Input: part model. Units: mm. Frame: model coordinates. A direction names the side the tool comes from. Give positions to 0.01 mm unless a question says otherwise; leave off trailing zeros. Write each loop counter-clockwise with the first axis right and the second up, starting at its lowest first coordinate (ties: lowest second). Pieces come first, ordered by that corner, then holes. Notation, with made-up numbers: (-23, 21) - (-12, 21) arc R17 cw to (-12, 41) - close; hole circle Ø6 at (27.25, -37). An arc over 180 degrees is marked (long way). Answer as CSV lines item,"result".
```python
from build123d import *

# Parameters (mm, degrees)
SKETCH1_W                 = 90
SKETCH1_H                 = 72
BOSS_EXTRUDE1_DEPTH       = 40
SHELL1_T                  = -2
SHELL1_THICKNESS_2_FACE_W = 86
SHELL1_THICKNESS_2_FACE_H = 38
SHELL1_THICKNESS_2_DEPTH  = 1
SHELL1_THICKNESS_3_FACE_W = 86
SHELL1_THICKNESS_3_FACE_H = 38
SHELL1_THICKNESS_3_DEPTH  = 1
SHELL1_THICKNESS_4_FACE_W = 66
SHELL1_THICKNESS_4_FACE_H = 38
SHELL1_THICKNESS_4_DEPTH  = 1.5
SKETCH2_R                 = 1.5
CUT_EXTRUDE1_DEPTH        = 2
CUT_EXTRUDE2_DEPTH        = 88
BOSS_EXTRUDE2_REACH       = 103.874
SKETCH4_W                 = 2
SKETCH4_H                 = 5
SKETCH5_R                 = 1.65
SKETCH5_W                 = 45
SKETCH5_H                 = 15
CUT_EXTRUDE3_DEPTH        = 3.5
CUT_EXTRUDE4_DEPTH        = 2.1
CUT_EXTRUDE5_REACH        = 106.862
SKETCH7_R                 = 2.55
SKETCH7_W                 = 10
SKETCH7_H                 = 10
SKETCH8_W                 = 16
SKETCH8_H                 = 9
SKETCH8_W_2               = 11
SKETCH8_H_2               = 7
CUT_EXTRUDE6_DEPTH        = 3
BOSS_EXTRUDE3_DEPTH       = 70
SKETCH10_R                = 1.65
SKETCH10_W                = 15.5
SKETCH10_H                = 9.5
CUT_EXTRUDE7_DEPTH        = 3
CUT_EXTRUDE8_DEPTH        = 2.1
FILLET3_R                 = 1
FILLET4_R                 = 0.5
FILLET5_R                 = 0.5
FILLET6_R                 = 0.5
FILLET7_R                 = 6
FILLET8_R                 = 4
FILLET9_R                 = 2
FILLET10_R                = 2


with BuildPart() as part:
    # Sketch1 → Boss-Extrude1 (new body)
    with BuildSketch(Plane(origin=(0, 0, 0), x_dir=(1, 0, 0), z_dir=(0, 1, 0))):
        Rectangle(SKETCH1_W, SKETCH1_H)
    extrude(amount=BOSS_EXTRUDE1_DEPTH)

    # Shell1
    shell1_openings = [part.faces().sort_by_distance(p)[0] for p in [
        (0, 40, 0),
    ]]
    offset(amount=SHELL1_T, openings=shell1_openings, kind=Kind.INTERSECTION)

    # Shell1 thickness 2 face (on inner face of the shell) → Shell1 thickness 2 (add)
    with BuildSketch(Plane(origin=(0, 21, 34), x_dir=(1, 0, 0), z_dir=(0, 0, 1))):
        Rectangle(SHELL1_THICKNESS_2_FACE_W, SHELL1_THICKNESS_2_FACE_H)
    extrude(amount=-SHELL1_THICKNESS_2_DEPTH)

    # Shell1 thickness 3 face (on inner face of the shell) → Shell1 thickness 3 (add)
    with BuildSketch(Plane(origin=(0, 21, -34), x_dir=(-1, 0, 0), z_dir=(0, 0, -1))):
        Rectangle(SHELL1_THICKNESS_3_FACE_W, SHELL1_THICKNESS_3_FACE_H)
    extrude(amount=-SHELL1_THICKNESS_3_DEPTH)

    # Shell1 thickness 4 face (on inner face of the shell) → Shell1 thickness 4 (add)
    with BuildSketch(Plane(origin=(43, 21, 0), x_dir=(0, 0, 1), z_dir=(1, 0, 0))):
        Rectangle(SHELL1_THICKNESS_4_FACE_W, SHELL1_THICKNESS_4_FACE_H)
    extrude(amount=-SHELL1_THICKNESS_4_DEPTH)

    # Sketch2 → Cut-Extrude1 (cut)
    with BuildSketch(Plane(origin=(0, 2, 0), x_dir=(1, 0, 0), z_dir=(0, 1, 0))):
        with Locations(Location((37.5, 27.5, 0), (0, 0, 270))):
            Circle(SKETCH2_R)
        with Locations(Location((-37.5, 27.5, 0), (0, 0, 270))):
            Circle(SKETCH2_R)
        with Locations(Location((-37.5, -27.5, 0), (0, 0, 270))):
            Circle(SKETCH2_R)
        with Locations(Location((37.5, -27.5, 0), (0, 0, 270))):
            Circle(SKETCH2_R)
    extrude(amount=-CUT_EXTRUDE1_DEPTH, mode=Mode.SUBTRACT)

    # Sketch3 → Cut-Extrude2 (cut)
    with BuildSketch(Plane(origin=(45, 0, 0), x_dir=(0, 0, -1), z_dir=(1, 0, 0))):
        Polygon((-30.5, 40), (-33.5, 37), (33.5, 37), (30.5, 40), align=None)
    extrude(amount=-CUT_EXTRUDE2_DEPTH, mode=Mode.SUBTRACT)

    # Sketch4 → Boss-Extrude2 (add, up to next)
    with BuildSketch(Plane.ZY.offset(-41.5), mode=Mode.PRIVATE) as boss_extrude2_sk1:
        Polygon((30.5, 40), (33, 37.5), (33, 40), align=None)
    boss_extrude2_tool1 = extrude(boss_extrude2_sk1.sketch, amount=BOSS_EXTRUDE2_REACH, mode=Mode.PRIVATE) - part.part
    # Sketch4 → Boss-Extrude2 (add, up to next)
    with BuildSketch(Plane.ZY.offset(-41.5), mode=Mode.PRIVATE) as boss_extrude2_sk2:
        Polygon((-33, 37.5), (-30.5, 40), (-33, 40), align=None)
    boss_extrude2_tool2 = extrude(boss_extrude2_sk2.sketch, amount=BOSS_EXTRUDE2_REACH, mode=Mode.PRIVATE) - part.part
    # Sketch4 → Boss-Extrude2 (add, up to next)
    with BuildSketch(Plane.ZY.offset(-41.5), mode=Mode.PRIVATE) as boss_extrude2_sk3:
        with Locations((-32, 34.5)):
            Rectangle(SKETCH4_W, SKETCH4_H)
    boss_extrude2_tool3 = extrude(boss_extrude2_sk3.sketch, amount=BOSS_EXTRUDE2_REACH, mode=Mode.PRIVATE) - part.part
    # Sketch4 → Boss-Extrude2 (add, up to next)
    with BuildSketch(Plane.ZY.offset(-41.5), mode=Mode.PRIVATE) as boss_extrude2_sk4:
        with Locations((32, 34.5)):
            Rectangle(SKETCH4_W, SKETCH4_H)
    boss_extrude2_tool4 = extrude(boss_extrude2_sk4.sketch, amount=BOSS_EXTRUDE2_REACH, mode=Mode.PRIVATE) - part.part
    add(boss_extrude2_tool1.solids().sort_by_distance((41.5, 39.166667, 32.166667))[0])
    add(boss_extrude2_tool2.solids().sort_by_distance((41.5, 39.166667, -32.166667))[0])
    add(boss_extrude2_tool3.solids().sort_by_distance((41.5, 34.5, -32))[0])
    add(boss_extrude2_tool4.solids().sort_by_distance((41.5, 34.5, 32))[0])

    # Sketch5 → Cut-Extrude3 (cut)
    with BuildSketch(Plane(origin=(45, 0, 0), x_dir=(0, 0, -1), z_dir=(1, 0, 0))):
        with Locations((0, 17)):
            Circle(SKETCH5_R)
        with Locations((0, 29.5)):
            Rectangle(SKETCH5_W, SKETCH5_H)
    extrude(amount=-CUT_EXTRUDE3_DEPTH, mode=Mode.SUBTRACT)

    # Sketch6 → Cut-Extrude4 (cut)
    with BuildSketch(Plane.ZY.offset(-41.5)):
        Polygon((3.117691454, 17), (1.558845727, 19.7), (-1.558845727, 19.7), (-3.117691454, 17), (-1.558845727, 14.3), (1.558845727, 14.3), align=None)
    extrude(amount=-CUT_EXTRUDE4_DEPTH, mode=Mode.SUBTRACT)

    # Sketch7 → Cut-Extrude5 (cut, up to next)
    with BuildSketch(Plane.ZY.offset(45), mode=Mode.PRIVATE) as cut_extrude5_sk1:
        with Locations((-22.5, 30)):
            Circle(SKETCH7_R)
    cut_extrude5_tool1 = extrude(cut_extrude5_sk1.sketch, amount=-CUT_EXTRUDE5_REACH, mode=Mode.PRIVATE) & part.part
    # Sketch7 → Cut-Extrude5 (cut, up to next)
    with BuildSketch(Plane.ZY.offset(45), mode=Mode.PRIVATE) as cut_extrude5_sk2:
        with Locations((-7.5, 30)):
            Circle(SKETCH7_R)
    cut_extrude5_tool2 = extrude(cut_extrude5_sk2.sketch, amount=-CUT_EXTRUDE5_REACH, mode=Mode.PRIVATE) & part.part
    # Sketch7 → Cut-Extrude5 (cut, up to next)
    with BuildSketch(Plane.ZY.offset(45), mode=Mode.PRIVATE) as cut_extrude5_sk3:
        with Locations((7.5, 30)):
            Circle(SKETCH7_R)
    cut_extrude5_tool3 = extrude(cut_extrude5_sk3.sketch, amount=-CUT_EXTRUDE5_REACH, mode=Mode.PRIVATE) & part.part
    # Sketch7 → Cut-Extrude5 (cut, up to next)
    with BuildSketch(Plane.ZY.offset(45), mode=Mode.PRIVATE) as cut_extrude5_sk4:
        with Locations((22.5, 30)):
            Circle(SKETCH7_R)
    cut_extrude5_tool4 = extrude(cut_extrude5_sk4.sketch, amount=-CUT_EXTRUDE5_REACH, mode=Mode.PRIVATE) & part.part
    # Sketch7 → Cut-Extrude5 (cut, up to next)
    with BuildSketch(Plane.ZY.offset(45), mode=Mode.PRIVATE) as cut_extrude5_sk5:
        with Locations((-4, 17)):
            Rectangle(SKETCH7_W, SKETCH7_H)
    cut_extrude5_tool5 = extrude(cut_extrude5_sk5.sketch, amount=-CUT_EXTRUDE5_REACH, mode=Mode.PRIVATE) & part.part
    add(cut_extrude5_tool1.solids().sort_by_distance((-45, 30, -22.5))[0], mode=Mode.SUBTRACT)
    add(cut_extrude5_tool2.solids().sort_by_distance((-45, 30, -7.5))[0], mode=Mode.SUBTRACT)
    add(cut_extrude5_tool3.solids().sort_by_distance((-45, 30, 7.5))[0], mode=Mode.SUBTRACT)
    add(cut_extrude5_tool4.solids().sort_by_distance((-45, 30, 22.5))[0], mode=Mode.SUBTRACT)
    add(cut_extrude5_tool5.solids().sort_by_distance((-45, 17, -4))[0], mode=Mode.SUBTRACT)

    # Sketch8 → Cut-Extrude6 (cut)
    with BuildSketch(Plane.XY.offset(36)):
        with Locations((-17, 18)):
            Rectangle(SKETCH8_W, SKETCH8_H)
        with Locations((6.5, 18)):
            Rectangle(SKETCH8_W_2, SKETCH8_H_2)
    extrude(amount=-CUT_EXTRUDE6_DEPTH, mode=Mode.SUBTRACT)

    # Sketch9 → Boss-Extrude3 (add)
    with BuildSketch(Plane.XY.offset(-36)):
        Polygon((21.517157288, 0), (-21.517157288, 0), (-24.517157288, -3), (24.517157288, -3), align=None)
    extrude(amount=BOSS_EXTRUDE3_DEPTH)

    # Sketch10 → Cut-Extrude7 (cut)
    with BuildSketch(Plane(origin=(0, 0, -36), x_dir=(-1, 0, 0), z_dir=(0, 0, -1))):
        with Locations((0, 12)):
            Circle(SKETCH10_R)
        with Locations((0, 26.75)):
            Rectangle(SKETCH10_W, SKETCH10_H)
    extrude(amount=-CUT_EXTRUDE7_DEPTH, mode=Mode.SUBTRACT)

    # Sketch11 → Cut-Extrude8 (cut)
    with BuildSketch(Plane.XY.offset(-33)):
        Polygon((1.558845727, 14.7), (-1.558845727, 14.7), (-3.117691454, 12), (-1.558845727, 9.3), (1.558845727, 9.3), (3.117691454, 12), align=None)
    extrude(amount=-CUT_EXTRUDE8_DEPTH, mode=Mode.SUBTRACT)

    # Fillet3
    fillet3_edges = [part.edges().sort_by_distance(p)[0] for p in [
        (43.25, 37, 22.5),
        (43.25, 22, 22.5),
        (43.25, 22, -22.5),
        (43.25, 37, -22.5),
    ]]
    fillet(fillet3_edges, radius=FILLET3_R)

    # Fillet4
    fillet4_edges = [part.edges().sort_by_distance(p)[0] for p in [
        (-44, 22, -9),
        (-44, 12, -9),
        (-44, 12, 1),
        (-44, 22, 1),
    ]]
    fillet(fillet4_edges, radius=FILLET4_R)

    # Fillet5
    fillet5_edges = [part.edges().sort_by_distance(p)[0] for p in [
        (-25, 22.5, 34.5),
        (-25, 13.5, 34.5),
        (-9, 13.5, 34.5),
        (-9, 22.5, 34.5),
        (1, 21.5, 34.5),
        (1, 14.5, 34.5),
        (12, 14.5, 34.5),
        (12, 21.5, 34.5),
    ]]
    fillet(fillet5_edges, radius=FILLET5_R)

    # Fillet6
    fillet6_edges = [part.edges().sort_by_distance(p)[0] for p in [
        (7.75, 31.5, -34.5),
        (7.75, 22, -34.5),
        (-7.75, 22, -34.5),
        (-7.75, 31.5, -34.5),
    ]]
    fillet(fillet6_edges, radius=FILLET6_R)

    # Fillet7
    fillet7_edges = [part.edges().sort_by_distance(p)[0] for p in [
        (-43, 34.5, 31),
        (41.5, 34.5, 31),
        (-43, 34.5, -31),
        (41.5, 34.5, -31),
    ]]
    fillet(fillet7_edges, radius=FILLET7_R)

    # Fillet8
    fillet8_edges = [part.edges().sort_by_distance(p)[0] for p in [
        (41.5, 17, 33),
        (-43, 17, 33),
        (-43, 17, -33),
        (41.5, 17, -33),
    ]]
    fillet(fillet8_edges, radius=FILLET8_R)

    # Fillet9
    fillet9_edges = [part.edges().sort_by_distance(p)[0] for p in [
        (-0.75, 2, -33),
        (-43, 2, 0),
        (-0.75, 2, 33),
        (41.5, 2, 0),
        (-41.828427125, 2, 31.828427125),
        (40.328427125, 2, 31.828427125),
        (40.328427125, 2, -31.828427125),
        (-41.828427125, 2, -31.828427125),
    ]]
    fillet(fillet9_edges, radius=FILLET9_R)

    # Fillet10
    fillet10_edges = [part.edges().sort_by_distance(p)[0] for p in [
        (-45, 20, -36),
        (-45, 20, 36),
    ]]
    fillet(fillet10_edges, radius=FILLET10_R)


solid = part.part
```
Item 1: Ray query, line 1 (Y direction, x = 0, z = -35.55); line 2 (X direction, y = 36, z = 24.5); line 3 (Z direction, x = 15, y = 20). Return the intervals inside material, ascending. Write a range as from..to.
The answers:
line 1,"-3..10.35, 13.65..22, 31.5..40"
line 2,"-45..-43, 41.5..45"
line 3,"-36..-33, 33..36"
Item 2: Cut plane C-C on x = 33. Return the cut outline in (y, z).
The answers:
outline,"(0, -36) - (40, -36) - (40, -30.5) - (37, -33.5) - (37, -31) - (32, -31) - (32, -33) - (4, -33) arc R2 cw to (2, -31) - (2, 31) arc R2 cw to (4, 33) - (32, 33) - (32, 31) - (37, 31) - (37, 33.5) - (40, 30.5) - (40, 36) - (0, 36) - close"
Item 3: Mould query, pull axis X, two halves, no side actions, for faces 1 (the face through (-44.4, 20.28, 35.43)), 2 (the face through (-41.797, 18.196, 31.859)), 3 (the face through (43, 29, -22.5)), 4 (the face through (-43, 26, 0)). Classes: +X half, -X half, draft (parallel to the pull), parting line (faces both ways), or undercut.
The answers:
face 1,"-X half"
face 2,"undercut"
face 3,"draft"
face 4,"undercut"
Item 4: Cut plane D-D on z = 27.5. Return the cut outline in (x, y).
The answers:
outline,"(-45, 0) - (-39, 0) - (-39, 2) - (-41, 2) arc R2 cw to (-43, 4) - (-43, 32) - (-42.45, 32) - (-42.45, 37) - (-43, 37) - (-43, 40) - (-45, 40) - close; (-36, 0) - (-21.52, 0) - (-24.52, -3) - (24.52, -3) - (21.52, 0) - (36, 0) - (36, 2) - (-36, 2) - close; (39, 0) - (45, 0) - (45, 37) - (40.95, 37) - (40.95, 32) - (41.5, 32) - (41.5, 4) arc R2 cw to (39.5, 2) - (39, 2) - close"
Item 5: Cut plane B-B on x = 0. Count the separate pieces of the cut face and the enclosed holes in it, plus the area to 3 significant figures.
The answers:
separate pieces,"3"
enclosed holes,"0"
area,"567 mm²"
Item 6: Cut plane A-A on z = -7.5. Return the cut outline in (x, y), plus the area to 3 significant figures.
The answers:
outline,"(-45, 0) - (-21.52, 0) - (-24.52, -3) - (24.52, -3) - (21.52, 0) - (45, 0) - (45, 22) - (41.5, 22) - (41.5, 4) arc R2 cw to (39.5, 2) - (-41, 2) arc R2 cw to (-43, 4) - (-43, 12) - (-45, 12) - close; (-45, 22) - (-43, 22) - (-43, 27.45) - (-45, 27.45) - close; (-45, 32.55) - (-43, 32.55) - (-43, 40) - (-45, 40) - close"
area,"436 mm²"
Item 7: Reachability of faces 5 (the face through (6, 14.5, 35)), 6 (the face through (-2.327, 13.369, -34.035)), 7 (the face through (0, -3, -1)), 8 (the face through (0.4, 10.4, -35.6)) from +Z, -Z, +X, -X, +Y, -Y: full face, straight path, thin tool, end or side. Return the list, or none.
The answers:
face 5,"+Z"
face 6,"none"
face 7,"+Z, -Z, +X, -X, -Y"
face 8,"-Z"
Item 8: Contact query for flat-ended pins moving along their axis: pin 1 (6 mm diameter, centred on x = -32.5, z = -12.5, fed in from +Y); pin 2 (2.5 mm diameter, centred on y = 25, z = -35, fed in from -X); pin 3 (1.8 mm diameter, centred on x = 43.5, z = -0.5, fed in from +Y); pin 4 (2.5 mm diameter, centred on x = 42.5, z = 0.5, fed in from -Y). Output: stop coordinate, or through.
The answers:
pin 1,"y = 2"
pin 2,"x = -45"
pin 3,"y = 22"
pin 4,"y = 0"
